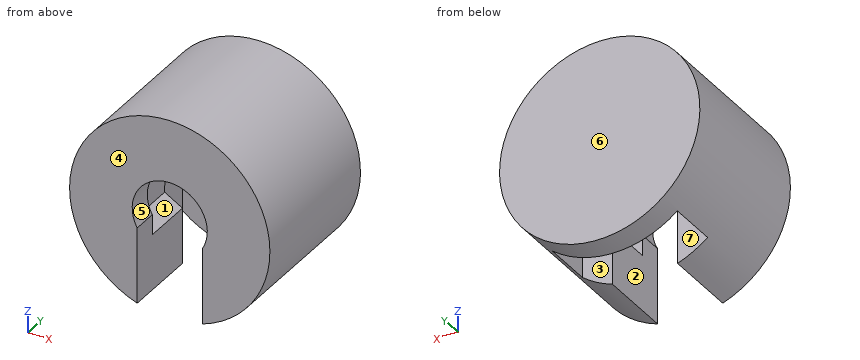
from build123d import *

# Parameters (mm, degrees)
SKETCH1_R           = 20
BOSS_EXTRUDE1_DEPTH = 10
CUT_EXTRUDE2_DEPTH  = 5
SKETCH5_R           = 20
BOSS_EXTRUDE3_DEPTH = 15
SKETCH6_R           = 20
BOSS_EXTRUDE4_DEPTH = 5
SKETCH7_R           = 7.5
CUT_EXTRUDE3_DEPTH  = 15
CUT_EXTRUDE4_DEPTH  = 42.231056256


with BuildPart() as part:
    # Sketch1 → Boss-Extrude1 (new body)
    with BuildSketch(Plane(origin=(0, 0, 0), x_dir=(1, 0, 0), z_dir=(0, 1, 0))):
        with Locations(Location((0, 0, 0), (0, 0, 270))):
            Circle(SKETCH1_R)
    extrude(amount=BOSS_EXTRUDE1_DEPTH)

    # Sketch2 → Cut-Extrude2 (cut)
    with BuildSketch(Plane(origin=(0, 10, 0), x_dir=(1, 0, 0), z_dir=(0, 1, 0))):
        Polygon((10.04843053, -5.688794004), (9.950855389, 5.857799105), (-0.097575141, 11.546593109), (-10.04843053, 5.688794004), (-9.950855389, -5.857799105), (0.097575141, -11.546593109), align=None)
    extrude(amount=-CUT_EXTRUDE2_DEPTH, mode=Mode.SUBTRACT)

    # Sketch5 → Boss-Extrude3 (add)
    with BuildSketch(Plane(origin=(0, 10, 0), x_dir=(1, 0, 0), z_dir=(0, 1, 0))):
        with Locations(Location((0, 0, 0), (0, 0, 270))):
            Circle(SKETCH5_R)
        Polygon((-9.950855389, -5.857799105), (0.097575141, -11.546593109), (10.04843053, -5.688794004), (9.950855389, 5.857799105), (-0.097575141, 11.546593109), (-10.04843053, 5.688794004), align=None, mode=Mode.SUBTRACT)
    extrude(amount=BOSS_EXTRUDE3_DEPTH)

    # Sketch6 → Boss-Extrude4 (add)
    with BuildSketch(Plane(origin=(0, 25, 0), x_dir=(1, 0, 0), z_dir=(0, 1, 0))):
        with Locations(Location((0, 0, 0), (0, 0, 270))):
            Circle(SKETCH6_R)
    extrude(amount=BOSS_EXTRUDE4_DEPTH)

    # Sketch7 → Cut-Extrude3 (cut)
    with BuildSketch(Plane.XZ):
        with Locations(Location((0, 0, 0), (0, 0, 270))):
            Circle(SKETCH7_R)
    extrude(amount=-CUT_EXTRUDE3_DEPTH, mode=Mode.SUBTRACT)

    # Sketch8 → Cut-Extrude4 (cut, through all)
    with BuildSketch(Plane.XY):
        Polygon((-6.5, 15), (-6.5, 0), (6.5, 0), (6.5, 15), (12.5, 15), (12.5, 25), (-12.5, 25), (-12.5, 15), align=None)
    extrude(amount=-CUT_EXTRUDE4_DEPTH, mode=Mode.SUBTRACT)


solid = part.part
Input: part model. Units: mm. Frame: model coordinates. Face numbers are marked on the shaded views. A direction names the side the tool comes from. Give positions to 0.01 mm unless a question says otherwise; leave off trailing zeros. Write each loop counter-clockwise with the first axis right and the second up, starting at its lowest first coordinate (ties: lowest second). Pieces come first, ordered by that corner, then holes. Notation, with made-up numbers: M -24.5,34 L -20.5,34 A17 cw -20.5,63 Z; hole C 83.5,45.5 d11. An arc over 180 degrees is marked long. Use one line per item in the form item = value.
1. Cut plane C-C on z = -15. Return loops of the section in (x, y).
Outcome:
outline = M -13.23,0 L -6.5,0 L -6.5,15 L -12.5,15 L -12.5,25 L 12.5,25 L 12.5,15 L 6.5,15 L 6.5,0 L 13.23,0 L 13.23,30 L -13.23,30 Z
2. Reachability of the marked faces 1, 2 and 3 from +Z, -Z, +X, -X, +Y, -Y: full face, straight path, thin tool, end or side. Return the list, or none.
Outcome:
face_1 = none
face_2 = -Z, -Y
face_3 = -Z
3. Cut plane B-B on x = -1.5. Return loops of the section in (y, z).
Outcome:
outline = M 0,7.35 L 5,7.35 L 5,10.64 L 25,10.64 L 25,-19.94 L 30,-19.94 L 30,19.94 L 0,19.94 Z
4. Cut plane D-D on y = 18. Return loops of the section in (x, z), and give its area (3 significant figures).
Outcome:
outline = M -12.5,-15.61 L -12.5,0 L -10,0 L -9.95,5.86 L 0.1,11.55 L 10.05,5.69 L 10,0 L 12.5,0 L 12.5,-15.61 A20 ccw long Z
area = 618 mm²
5. First-contact query: P1, Ø8, axis at x = -6.5, y = 16, coming from the -Z side; P2, Ø3, axis at y = 20.5, z = 6, coming from the +X side; P3, Ø7.5, axis at x = 1.5, z = -3, coming from the -Y side. Flat tips, straight axial feed; report the tip coordinate or a pass-through.
Outcome:
P1 = -18.91
P2 = 19.49
P3 = 25
6. Mould query, pull axis Y, two halves, no side actions, for the marked faces 4, 5, 6 and 7. Classes: released by +Y, released by -Y, zero draft, split by the parting line, or undercut.
Outcome:
face_4 = released by -Y
face_5 = zero draft
face_6 = released by +Y
face_7 = undercut
7. Ray query, L1, parallel to X at y = 2.65, z = 0; L2, parallel to Y at x = 10.5, z = -15; L3, parallel to X at y = 8.75, z = 1. Return the intervals inside material, ascending.
Outcome:
L1 = -20 to -7.5, 7.5 to 20
L2 = 0 to 15, 25 to 30
L3 = -19.97 to -9.99, 10.01 to 19.97
8. Cut plane A-A on y = 9.25. Return loops of the section in (x, z).
Outcome:
outline = M -10.05,-5.69 L -9.95,5.86 L 0.1,11.55 L 10.05,5.69 L 9.95,-5.86 L 6.5,-7.81 L 6.5,-18.91 A20 ccw long -6.5,-18.91 L -6.5,-7.78 Z
